```python
from build123d import *

# Parameters (mm, degrees)
SKETCH1_W           = 20.5
SKETCH1_H           = 37.6
SKETCH1_W_2         = 12.5
SKETCH1_H_2         = 23.6
BOSS_EXTRUDE1_DEPTH = 28
SKETCH2_R           = 1.92
CUT_EXTRUDE1_DEPTH  = 13
SKETCH3_W           = 8
SKETCH3_H           = 7
CUT_EXTRUDE2_DEPTH  = 8
SKETCH4_W           = 8
SKETCH4_H           = 7
CUT_EXTRUDE3_DEPTH  = 20


with BuildPart() as part:
    # Sketch1 → Boss-Extrude1 (new body)
    with BuildSketch(Plane(origin=(0, 0, 0), x_dir=(0, 0, -1), z_dir=(1, 0, 0))):
        with Locations((-0.15, -0.55)):
            Rectangle(SKETCH1_W, SKETCH1_H)
        with Locations((-0.15, -0.55)):
            Rectangle(SKETCH1_W_2, SKETCH1_H_2, mode=Mode.SUBTRACT)
    extrude(amount=BOSS_EXTRUDE1_DEPTH)

    # Sketch2 → Cut-Extrude1 (cut)
    with BuildSketch(Plane(origin=(28, 0, 0), x_dir=(0, 0, -1), z_dir=(1, 0, 0))):
        with Locations((0, 13.45)):
            Circle(SKETCH2_R)
    extrude(amount=-CUT_EXTRUDE1_DEPTH, mode=Mode.SUBTRACT)

    # Sketch3 → Cut-Extrude2 (cut)
    with BuildSketch(Plane(origin=(15, 0, 0), x_dir=(0, 0, -1), z_dir=(1, 0, 0))):
        with Locations((0, 14.75)):
            Rectangle(SKETCH3_W, SKETCH3_H)
    extrude(amount=CUT_EXTRUDE2_DEPTH, mode=Mode.SUBTRACT)

    # Sketch4 → Cut-Extrude3 (cut)
    with BuildSketch(Plane(origin=(28, 0, 0), x_dir=(0, 0, -1), z_dir=(1, 0, 0))):
        with Locations((0, -15.85)):
            Rectangle(SKETCH4_W, SKETCH4_H)
    extrude(amount=-CUT_EXTRUDE3_DEPTH, mode=Mode.SUBTRACT)


solid = part.part
```
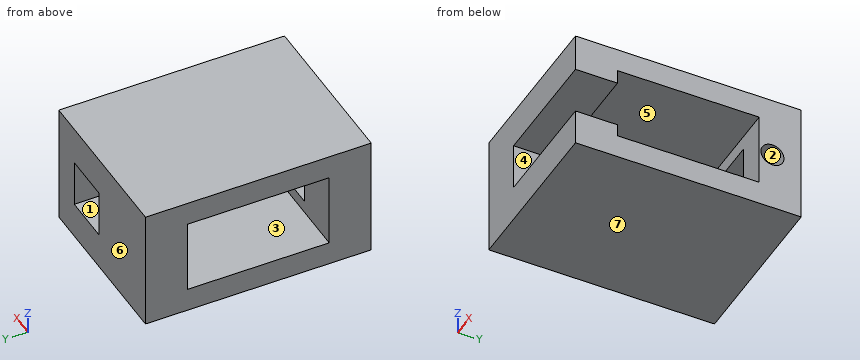
For this review, take the finished solid that the model builds, in its own axes (mm). Face numbers are marked on the shaded views. A direction names the side the tool comes from. Give positions to 0.01 mm unless a question says otherwise; leave off trailing zeros. Write each loop counter-clockwise with the first axis right and the second up, starting at its lowest first coordinate (ties: lowest second). Pieces come first, ordered by that corner, then holes. Notation, with made-up numbers: M 80.5,75.25 L 93.5,75.25 A37 cw 93.5,112.25 Z; hole C 6,22.5 d2. An arc over 180 degrees is marked long. One line per item, written item: value.
1) The part is to be moulded in two halves that separate along Y. For the marked faces 5, 6 and 7, say which applies: +Y half, -Y half, draft (parallel to the pull), parting line (faces both ways), or undercut.
Results are:
face 5: undercut
face 6: +Y half
face 7: draft
2) Take a section at C-C, the plane y = -0.5. Write out the cut boundary in (x, z), then the cut area to 3 significant figures.
Results are:
outline: M 0,-10.1 L 28,-10.1 L 28,-6.1 L 0,-6.1 Z; M 0,6.4 L 28,6.4 L 28,10.4 L 0,10.4 Z
area: 224 mm²
3) Take a section at B-B, the plane z = 0. Write out the cut boundary in (x, y), then the cut area to 3 significant figures.
Results are:
outline: M 0,-19.35 L 8,-19.35 L 8,-12.35 L 0,-12.35 Z; M 0,11.25 L 15,11.25 L 15,18.25 L 0,18.25 Z; M 23,11.25 L 28,11.25 L 28,11.53 L 23,11.53 Z; M 23,15.37 L 28,15.37 L 28,18.25 L 23,18.25 Z
area: 177 mm²
4) Take a section at D-D, the plane z = -2.5. Write out the cut boundary in (x, y).
Results are:
outline: M 0,-19.35 L 8,-19.35 L 8,-12.35 L 0,-12.35 Z; M 0,11.25 L 15,11.25 L 15,18.25 L 0,18.25 Z; M 23,11.25 L 28,11.25 L 28,18.25 L 23,18.25 Z
5) For line 1 (Z direction, x = 26, y = 5.5); line 2 (Y direction, x = 2.75, z = -2.25); line 3 (Y direction, x = 24.5, z = 0), list the stretches that pass through material, from the lowest coordinate up. Write a range as from..to.
Results are:
line 1: z = -10.1..-6.1, 6.4..10.4
line 2: y = -19.35..-12.35, 11.25..18.25
line 3: y = 11.25..11.53, 15.37..18.25
6) Take a section at A-A, the plane x = 17. Write out the cut boundary in (y, z), then the cut area to 3 significant figures.
Results are:
outline: M -19.35,-10.1 L 18.25,-10.1 L 18.25,-4 L 11.25,-4 L 11.25,-6.1 L -12.35,-6.1 L -12.35,-4 L -19.35,-4 Z; M -19.35,4 L -12.35,4 L -12.35,6.4 L 11.25,6.4 L 11.25,4 L 18.25,4 L 18.25,10.4 L -19.35,10.4 Z
area: 364 mm²
7) For the marked faces 1, 2, 3 and 4, list the 3-axis set-ups (+Z, -Z, +X, -X, +Y, -Y) from which the entire face can be reached by the end or side of a thin tool; tool diameter is ignored.
Results are:
face 1: +Y, -Y
face 2: +X
face 3: +X, -X
face 4: +X, -Y
